Could you check a few things on this model? Use its own coordinates, in mm. Face numbers are marked on the shaded views. A direction names the side the tool comes from. Give positions to 0.01 mm unless a question says otherwise; leave off trailing zeros. Loops run counter-clockwise (first coordinate to the right, second up) from the corner with the lowest first, then second, coordinate; pieces in that order, holes last. Notation, with made-up numbers: M -34,19.25 L 18,19.25 A8 ccw 18,31.25 Z; hole C 52.25,40 d8. An arc over 180 degrees is marked long. Answer in a Markdown table with one row per item. Add a question column.
1. If we section it at C-C on x = -40: List the corners of the cut face in (y, z) for me.
2. I need wall thicknesses on line 1 along Y through (x, z) = (0, 8.5); line 2 along Y through (x, z) = (0, 14.9); line 3 along X through (y, z) = (-27.5, 7.25). Which ranges of each line are inside material? Lowest first, please. Write a range as from..to.
3. Thinking about a two-plate mould opening in X: for the marked faces 1, 2 and 3, which applies, released by +X, released by -X, zero draft, split by the parting line, or undercut?
4. I'm going to push flat-ended pins straight in: pin 1 Ø6 at (x, z) = (-35.5, 5) entering from +Y; pin 2 Ø2 at (x, y) = (-24, -18) entering from -Z; pin 3 Ø4 at (y, z) = (8.5, 3.5) entering from -X. Where does each tip first touch, or does it pass through?
5. If we section it at D-D on z = 10.75: Count the separate pieces of the cut face and the enclosed holes in it, then the cut area to 3 significant figures.
6. If we section it at A-A on x = 0: List the corners of the cut face in (y, z) for me, then the cut area to 3 significant figures.
7. Which directions (+Z, -Z, +X, -X, +Y, -Y) give clear straight access to the entire face, cutting with the end or side of a thin tool? Please do the marked faces 4 and 5.
8. If we section it at B-B on y = -5: List the corners of the cut face in (x, z) for me, then the cut area to 3 significant figures.
```python
from build123d import *

# Parameters (mm, degrees)
SKETCH_1_R          = 45
SKETCH_1_R_2        = 35
EXTRUDE_1_DEPTH     = 12
SKETCH_2_R          = 45
SKETCH_2_R_2        = 29
EXTRUDE_2_DEPTH     = 6
SKETCH_4_R          = 2
CUT_EXTRUDE_1_DEPTH = 18


with BuildPart() as part:
    # 草图1 → 凸台-拉伸1 (new body)
    with BuildSketch(Plane.XY):
        Circle(SKETCH_1_R)
        Circle(SKETCH_1_R_2, mode=Mode.SUBTRACT)
    extrude(amount=EXTRUDE_1_DEPTH)

    # 草图2 → 凸台-拉伸2 (add)
    with BuildSketch(Plane.XY.offset(12)):
        Circle(SKETCH_2_R)
        Circle(SKETCH_2_R_2, mode=Mode.SUBTRACT)
    extrude(amount=EXTRUDE_2_DEPTH)

    # 草图4 → 切除-拉伸1 (cut)
    with BuildSketch(Plane.XY.offset(18)):
        with Locations((0, 40)):
            Circle(SKETCH_4_R)
        with Locations((28.284271247, 28.284271247)):
            Circle(SKETCH_4_R)
        with Locations((40, 0)):
            Circle(SKETCH_4_R)
        with Locations((28.284271247, -28.284271247)):
            Circle(SKETCH_4_R)
        with Locations((0, -40)):
            Circle(SKETCH_4_R)
        with Locations((-28.284271247, -28.284271247)):
            Circle(SKETCH_4_R)
        with Locations((-40, 0)):
            Circle(SKETCH_4_R)
        with Locations((-28.284271247, 28.284271247)):
            Circle(SKETCH_4_R)
    extrude(amount=-CUT_EXTRUDE_1_DEPTH, mode=Mode.SUBTRACT)


solid = part.part
```
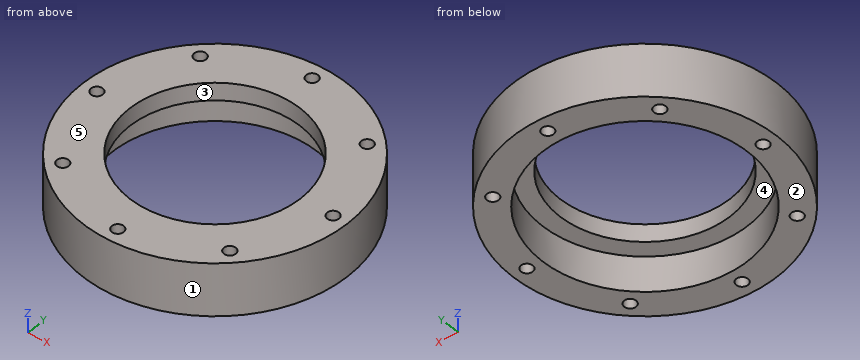
Results:
| question | item | result |
|---|---|---|
| 1 | outline | M -20.62,0 L -2,0 L -2,18 L -20.62,18 Z; M 2,0 L 20.62,0 L 20.62,18 L 2,18 Z |
| 2 | line 1 | -45..-42, -38..-35, 35..38, 42..45 |
| 2 | line 2 | -45..-42, -38..-29, 29..38, 42..45 |
| 2 | line 3 | -35.62..-30.12, -26.44..-21.65, 21.65..26.44, 30.12..35.62 |
| 3 | face 1 | split by the parting line |
| 3 | face 2 | zero draft |
| 3 | face 3 | undercut |
| 4 | pin 1 | y = 31.12 |
| 4 | pin 2 | z = 12 |
| 4 | pin 3 | x = -44.53 |
| 5 | separate pieces | 1 |
| 5 | enclosed holes | 9 |
| 5 | area | 2,410 mm2 |
| 6 | outline | M -45,0 L -42,0 L -42,18 L -45,18 Z; M -38,0 L -35,0 L -35,12 L -29,12 L -29,18 L -38,18 Z; M 29,12 L 35,12 L 35,0 L 38,0 L 38,18 L 29,18 Z; M 42,0 L 45,0 L 45,18 L 42,18 Z |
| 6 | area | 288 mm2 |
| 7 | face 4 | -Z |
| 7 | face 5 | +Z, +X, -X, +Y, -Y |
| 8 | outline | M -44.72,0 L -34.64,0 L -34.64,12 L -28.57,12 L -28.57,18 L -44.72,18 Z; M 28.57,12 L 34.64,12 L 34.64,0 L 44.72,0 L 44.72,18 L 28.57,18 Z |
| 8 | area | 436 mm2 |
